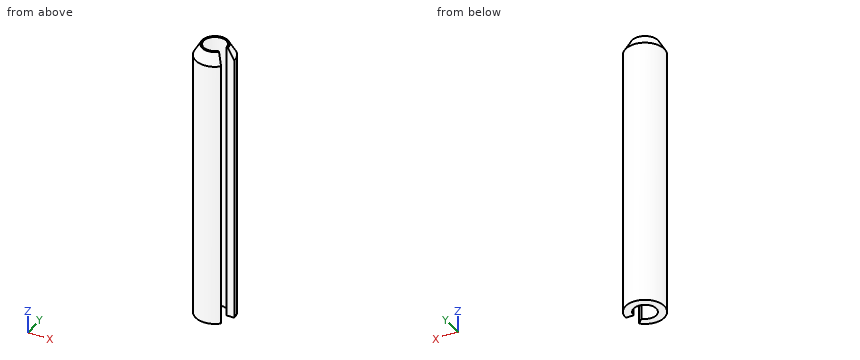
from build123d import *

# Parameters (mm, degrees)
F1_DEPTH = 21.75
F2_SIZE2 = 1.7320508076
F2_SIZE  = 1


with BuildPart() as f1:
    # F0 (on Top) → F1 (new body, symmetric)
    with BuildSketch(Plane.XY):
        with BuildLine():
            Line((1.75, 0), (3, 0))
            ThreePointArc((3, 0), (-2.7716385975, 1.1480502971), (2.1213203436, -2.1213203436))
            Line((2.1213203436, -2.1213203436), (1.2374368671, -1.2374368671))
            ThreePointArc((1.2374368671, -1.2374368671), (-1.6167891819, 0.6696960066), (1.75, 0))
        make_face()
    extrude(amount=F1_DEPTH, both=True)

    # F2
    f2_edges = [f1.edges().sort_by_distance(p)[0] for p in [
        (-2.771639, 1.14805, 21.75),
    ]]
    f2_side = f1.faces().sort_by_distance((-1.695183, 0.702168, 21.75))[0]
    chamfer(f2_edges, length=F2_SIZE, length2=F2_SIZE2, reference=f2_side)


solid = f1.part
The model under review builds one solid part; all positions refer to its coordinate system, in mm. Coordinates: 2 decimals unless noted, no trailing zeros. Loops run counter-clockwise (first coordinate to the right, second up) from the corner with the lowest first, then second, coordinate; pieces in that order, holes last. Notation, with made-up numbers: M 52.25,-28.75 L 107.25,-28.75 A32 cw 107.25,8.25 Z; hole C 10.25,55 d5. An arc over 180 degrees is marked long. Put each result on its own line as item: value. Start each with the question number.
Q1. Add section A-A (x = 0). Write out the cut boundary in (y, z).
Q2. Wall thickness on line 1 (Y direction, x = 0, z = -9); line 2 (Y direction, x = 1.25, z = 2); line 3 (X direction, y = 1, z = -1): over which ranges is each line inside the solid? List them lowest first.
Q3. Add section B-B (z = 9). Write out the cut boundary in (x, y), and give its area (3 significant figures).
Q4. Clearance check with flat-ended pins moving along their axes: pin 1 (1 mm diameter, centred on x = 2.5, z = 3.5, fed in from -Y); pin 2 (1.5 mm diameter, centred on y = 1.5, z = 1.5, fed in from +X). State where each tip first meets the part, or that it passes through.
Answers:
1. outline: M -3,-21.75 L -1.75,-21.75 L -1.75,21.75 L -2,21.75 L -3,20.02 Z; M 1.75,-21.75 L 3,-21.75 L 3,20.02 L 2,21.75 L 1.75,21.75 Z
2. line 1: y = -3 to -1.75, 1.75 to 3
2. line 2: y = -2.73 to -1.25, 1.22 to 2.73
2. line 3: x = -2.83 to -1.44, 1.44 to 2.83
3. outline: M 1.24,-1.24 A1.75 cw long 1.75,0 L 3,0 A3 ccw long 2.12,-2.12 Z
3. area: 16.3 mm^2
4. pin 1: stops at y = -2.24
4. pin 2: stops at x = 2.9
